Autodesk Inventor part; units mm, degrees
ref_plane "YZ Plane" through (0, 0, 0) normal (1, 0, 0) x (0, 1, 0)
ref_plane "XZ Plane" through (0, 0, 0) normal (0, 1, 0) x (-1, 0, 0)
ref_plane "XY Plane" through (0, 0, 0) normal (0, 0, 1) x (1, 0, 0)
sketch "Эскиз1" plane through (0, 0, 0) normal (0, 1, 0) x (-1, 0, 0)
  line L0 (-5, 11.7093) -> (-5, -48.2907)
  line L1 (15, 10.2093) -> (15, -46.7907)
  line L2 (15, 10.2093) -> (15, 14.2093)
  line L3 (15, -46.7907) -> (15, -50.7907)
  line L4 (15, 14.2093) -> (-5, 11.7093)
  line L5 (15, -50.7907) -> (-5, -48.2907)
  point P0 (0, 0)
  dimension "d0" = 60
  dimension "d3" = 20
  dimension "d4" = 4
  dimension "d5" = 4
extrude "Выдавливание1" add sketch "Эскиз1" along normal blind 2
fillet "Сопряжение1" radius 3 2 edges at (5, 1, -48.2907) (5, 1, 11.7093)
sketch "Эскиз3" plane through (0, 2, 0) normal (0, 1, 0) x (1, 0, 0)
  arc A0 (5, 45.6424) -> (2.3721, 48.6192) centre (2, 45.6424) ccw
  line L0 (5, 45.6424) -> (-10, 45.6424)
  line L1 (-10, 45.6424) -> (-10, 43.6424)
  line L2 (-10, 43.6424) -> (5, 43.6424)
  line L3 (5, 43.6424) -> (5, 45.6424)
  line L4 (5, -9.0609) -> (5, 45.6424)
  line L5 (5, 24.6424) -> (-10, 24.6424)
  line L6 (-10, 24.6424) -> (-10, 22.6424)
  line L7 (-10, 22.6424) -> (5, 22.6424)
  line L8 (5, 22.6424) -> (5, 24.6424)
  point P0 (0, 0)
  dimension "d21" = 15
  dimension "d22" = 2
  dimension "d23" = 2
  dimension "d24" = 19
extrude "Выдавливание2" add sketch "Эскиз3" along normal blind 7
fillet "Сопряжение2" radius 1 4 edges at (5, 5.5, -43.6424) (5, 5.5, -24.6424) (-10, 5.5, -43.6424) (-10, 5.5, -24.6424)
chamfer "Фаска1" distance 1 angle 45 1 edges at (-2.5, 2, -45.6424)
sketch "Эскиз4" plane through (0, 2, 0) normal (0, 1, 0) x (1, 0, 0)
  line L0 (5, -9.0609) -> (5, 45.6424)
  line L1 (5, 19.6424) -> (-15, 19.6424)
  line L2 (-15, 19.6424) -> (-15, 0.5424)
  line L3 (-15, 0.5424) -> (5, 0.5424)
  line L4 (5, 0.5424) -> (5, 19.6424)
  line L5 (-9, 43.6424) -> (4, 43.6424)
  point P0 (0, 0)
  point P1 (5, 0.5424)
  dimension "d31" = 20
  dimension "d32" = 19.1
  dimension "d33" = 24
extrude "Выдавливание3" add sketch "Эскиз4" along normal blind 4
sketch "Эскиз5" plane through (0, 6, 0) normal (0, 1, 0) x (1, 0, 0)
  line L0 (-15, 0.5424) -> (5, 0.5424)
  line L1 (-15, 19.6424) -> (5, 19.6424)
  line L2 (5, 0.5424) -> (-2, 0.5424)
  line L3 (-2, 0.5424) -> (-2, 19.6424)
  line L4 (-2, 19.6424) -> (5, 19.6424)
  line L5 (5, 19.6424) -> (5, 0.5424)
  point P0 (0, 0)
  point P1 (5, 19.6424)
  dimension "d36" = 7
extrude "Выдавливание4" cut sketch "Эскиз5" against normal blind 4
sketch "Эскиз6" plane through (0, 6, 0) normal (0, 1, 0) x (1, 0, 0)
  line L0 (-15, 50.7907) -> (-15, -14.2093)
  line L1 (-15, 0.5424) -> (-2, 0.5424)
  line L2 (-15, 1.7424) -> (-2, 1.7424)
  line L3 (-2, 1.7424) -> (-2, 0.5424)
  line L4 (-2, 0.5424) -> (-15, 0.5424)
  line L5 (-15, 0.5424) -> (-15, 1.7424)
  line L6 (-2, 0.5424) -> (-2, 19.6424)
  line L7 (-2, 19.6424) -> (-15, 19.6424)
  line L8 (-15, 19.6424) -> (-15, 18.4424)
  line L9 (-15, 18.4424) -> (-2, 18.4424)
  line L10 (-2, 18.4424) -> (-2, 19.6424)
  point P0 (0, 0)
  point P1 (-2, 18.4424)
  point P2 (-15, 19.6424)
  dimension "d39" = 1.2
  dimension "d40" = 1.2
extrude "Выдавливание5" cut sketch "Эскиз6" against normal blind 1 contours L7 L6 L9 L0 | L2 L3 L1 L0
fillet "Сопряжение3" radius 0.5 2 edges at (-8.5, 6, -1.7424) (-8.5, 6, -18.4424)
sketch "Эскиз7" plane through (0, 2, 0) normal (0, 1, 0) x (1, 0, 0)
  line L0 (-15, -9.8754) -> (-6, -9.8754)
  line L1 (-6, -9.8754) -> (-6, -7.8754)
  line L2 (-6, -7.8754) -> (-15, -7.8754)
  line L3 (-15, -7.8754) -> (-15, -9.8754)
  line L4 (-15, 0.5424) -> (-15, -14.2093)
  line L5 (-6, -2.2754) -> (-15, -2.2754)
  line L6 (-15, -2.2754) -> (-15, -4.2754)
  line L7 (-15, -4.2754) -> (-6, -4.2754)
  line L8 (-6, -4.2754) -> (-6, -2.2754)
  point P0 (0, 0)
  dimension "d44" = 2
  dimension "d45" = 0
  dimension "d46" = 9
  dimension "d47" = 2
  dimension "d48" = 3.6
extrude "Выдавливание6" add sketch "Эскиз7" along normal blind 15.3
fillet "Сопряжение4" radius 0.5 8 edges at (-6, 17.3, 3.2754) (-10.5, 17.3, 4.2754) (-10.5, 17.3, 7.8754) (-6, 17.3, 8.8754) (-6, 9.65, 4.2754) (-6, 9.65, 7.8754) (-15, 9.65, 4.2754) (-15, 9.65, 7.8754)
chamfer "Фаска2" distance 1 angle 45 3 edges at (-10.5, 2, 9.8754) (-10.5, 2, 2.2754) (-2.5, 2, -22.6424)
properties part number "ploh"
Geometry: final body of the model. Coordinates: model frame, mm. A direction names the side the tool comes from. Coordinates: 2 decimals unless noted, no trailing zeros. Order: outer loops, then holes, each group sorted by start corner. A loop starts at its lowest first (then second) coordinate and runs counter-clockwise, first axis right, second up. Notation, with made-up numbers: (43, 67) - (101, 67) arc R34 cw to (101, 101) - close; hole circle Ø11 at (-36.75, 42.25). An arc over 180 degrees is marked (long way). Return JSON: item names as keys, results as strings. Group by question number.
1. Material intervals for line 1 along Z through (x, y) = (-3.5, 3.5); line 2 along Z through (x, y) = (-1, 3.5); line 3 along Z through (x, y) = (-10.5, 8.5), sorted ascending. Write a range as [from, to].
2. Cut plane C-C (y = 1.25). Output: boundary loops of the cut face in (x, z), plus the area to 3 significant figures.
3. Pull-direction query (Z, two-part tool) for faces 4 (the face through (4.2, 1, 11.1)), 5 (the face through (-3, 5, -43.642)), 6 (the face through (-2, 6, -45.642)), 7 (the face through (5, 1, -18)); classes: pulls with the +Z half, pulls with the -Z half, needs draft (parallel to the pull), parting line crosses it, or undercut.
4. Cut plane A-A (y = 11.75). Output: boundary loops of the cut face in (x, z), plus the area to 3 significant figures.
5. Cut plane B-B (x = -10.75). Output: boundary loops of the cut face in (y, z).
6. Cut plane D-D (z = -34.5). Output: boundary loops of the cut face in (x, y).
7. Set-up query: faces 1 (the face through (-11, 10, 9.875)), 2 (the face through (-9, 5, -19)), 3 (the face through (-10, 5, -45)). Return all of +Z, -Z, +X, -X, +Y, -Y with unobstructed straight access to the full face (end or side cutting, diameter ignored); none if empty.
8. Pin query (flat end, axial travel): pin 1 (1.6 mm diameter, centred on x = -4.5, z = -23.5, fed in from +Y); pin 2 (3 mm diameter, centred on y = 10.5, z = 2, fed in from +X); pin 3 (6.5 mm diameter, centred on x = -9, y = 8, fed in from +Z). Return the tip coordinate at first contact, or that it passes through.
Resolved:
{
 "1": {"line 1": "z = [-45.64, -43.64], [-24.64, -22.64], [-19.64, -0.54]", "line 2": "z = [-45.64, -43.64], [-24.64, -22.64]", "line 3": "z = [2.28, 4.28], [7.88, 9.88]"},
 "2": {"outline": "(-15, -50.79) - (2.37, -48.62) arc R3 ccw to (5, -45.64) - (5, 9.06) arc R3 ccw to (2.37, 12.04) - (-15, 14.21) - close", "area": "1,250 mm²"},
 "3": {"face 4": "pulls with the +Z half", "face 5": "undercut", "face 6": "pulls with the -Z half", "face 7": "needs draft"},
 "4": {"outline": "(-15, 2.28) - (-6, 2.28) - (-6, 3.78) arc R0.5 ccw to (-6.5, 4.28) - (-14.5, 4.28) arc R0.5 ccw to (-15, 3.78) - close; (-15, 8.38) arc R0.5 ccw to (-14.5, 7.88) - (-6.5, 7.88) arc R0.5 ccw to (-6, 8.38) - (-6, 9.88) - (-15, 9.88) - close", "area": "35.8 mm²"},
 "5": {"outline": "(0, -50.26) - (2, -50.26) - (2, -19.64) - (5, -19.64) - (5, -18.44) - (5.5, -18.44) arc R0.5 ccw to (6, -17.94) - (6, -2.24) arc R0.5 ccw to (5.5, -1.74) - (5, -1.74) - (5, -0.54) - (2, -0.54) - (2, 1.28) - (3, 2.28) - (17.3, 2.28) - (17.3, 3.78) arc R0.5 ccw to (16.8, 4.28) - (2, 4.28) - (2, 7.88) - (16.8, 7.88) arc R0.5 ccw to (17.3, 8.38) - (17.3, 9.88) - (3, 9.88) - (2, 10.88) - (2, 13.68) - (0, 13.68) - close"},
 "6": {"outline": "(-15, 0) - (5, 0) - (5, 2) - (-15, 2) - close"},
 "7": {"face 1": "+Z, +X, -X, +Y", "face 2": "+X, -X, +Y", "face 3": "-Z, -X, +Y"},
 "8": {"pin 1": "stops at y = 9", "pin 2": "stops at x = -6", "pin 3": "stops at z = 9.88"}
}
